Input: part model. Units: mm. Frame: model coordinates. Face numbers are marked on the shaded views. A direction names the side the tool comes from. Coordinates: 2 decimals unless noted, no trailing zeros. Loops run counter-clockwise (first coordinate to the right, second up) from the corner with the lowest first, then second, coordinate; pieces in that order, holes last. Notation, with made-up numbers: M -12,49 L 22,49 A28 ccw 22,76 Z; hole C 72,7 d7. An arc over 180 degrees is marked long. Use a Markdown table: item, result. Add a question column.
1. Line query: L1, parallel to Y at x = 21, z = 0; L2, parallel to Y at x = -31, z = -14; L3, parallel to Y at x = -2.5, z = 23.5. Output: solid intervals per line, ascending. Write a range as [from, to].
2. Draft query along Y for the marked faces 1, 2, 3 and 4. Return one class per face: +Y half, -Y half, draft (parallel to the pull), parting line (faces both ways), or undercut.
3. Set-up query: the marked faces 5 and 6. Return all of +Z, -Z, +X, -X, +Y, -Y with unobstructed straight access to the full face (end or side cutting, diameter ignored); none if empty.
4. Pin query (flat end, axial travel): pin 1 (1.5 mm diameter, centred on y = -3.5, z = -18.5, fed in from +X); pin 2 (4 mm diameter, centred on y = -24, z = 32, fed in from -X); pin 3 (10 mm diameter, centred on x = 6.5, y = 18.5, fed in from -Z). Return the tip coordinate at first contact, or that it passes through.
5. Section A-A on y = -14.5. Output: boundary loops of the cut face in (x, z).
6. Section C-C on x = -25.5. State how many separate pieces and enclosed holes the cut face has, then the cut area to 3 significant figures.
7. Section D-D on y = 6. Output: boundary loops of the cut face in (x, z), then the cut area to 3 significant figures.
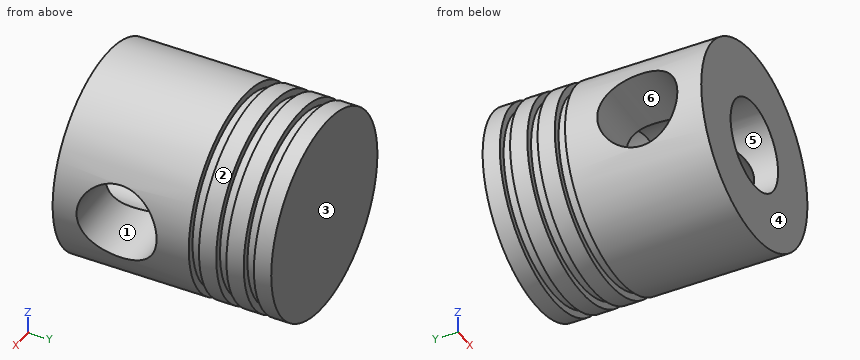
```python
from build123d import *

# Parameters (mm, degrees)
SKETCH4_R          = 16.9
CUT_EXTRUDE1_DEPTH = 42.5
SKETCH5_W          = 36
SKETCH5_H          = 40
SKETCH6_R          = 19
CUT_EXTRUDE2_DEPTH = 45


with BuildPart() as part:
    # Sketch2 → Revolve1 (revolve)
    with BuildSketch(Plane(origin=(0, 0, 0), x_dir=(0, 0, -1), z_dir=(1, 0, 0))):
        Polygon((39.5, 25.428946917), (39.5, 21.128946917), (42.5, 21.128946917), (42.5, 13.828946917), (39.5, 13.828946917), (39.5, 9.528946917), (42.5, 9.528946917), (42.5, -47.971053083), (0, -47.971053083), (0, 44.328946917), (42.5, 44.328946917), (42.5, 37.028946917), (39.5, 37.028946917), (39.5, 32.728946917), (42.5, 32.728946917), (42.5, 25.428946917), align=None)
    revolve(axis=Axis((0, -52.221053083, 0), (0, 1, 0)))

    # Sketch4 → Cut-Extrude1 (cut, symmetric)
    with BuildSketch(Plane(origin=(0, 0, 0), x_dir=(0, 0, -1), z_dir=(1, 0, 0))):
        with Locations((0, -20.971053083)):
            Circle(SKETCH4_R)
    extrude(amount=CUT_EXTRUDE1_DEPTH, both=True, mode=Mode.SUBTRACT)

    # Sketch5 → Cut-Revolve1 (revolve, cut)
    with BuildSketch(Plane(origin=(0, 0, 0), x_dir=(0, 0, -1), z_dir=(1, 0, 0))):
        with Locations((-18, 17.028946917)):
            Rectangle(SKETCH5_W, SKETCH5_H)
    revolve(axis=Axis((0, -52.221053083, 0), (0, 1, 0)), mode=Mode.SUBTRACT)

    # Sketch6 → Cut-Extrude2 (cut)
    with BuildSketch(Plane.XZ.offset(47.971053083)):
        Circle(SKETCH6_R)
    extrude(amount=-CUT_EXTRUDE2_DEPTH, mode=Mode.SUBTRACT)


solid = part.part
```
Answers below:
| question | item | result |
|---|---|---|
| 1 | L1 | y = [-47.97, -37.87], [-4.07, -2.97], [37.03, 44.33] |
| 1 | L2 | y = [-47.97, -30.44], [-11.5, -2.97], [37.03, 44.33] |
| 1 | L3 | y = [-47.97, -2.97], [37.03, 44.33] |
| 2 | face 1 | undercut |
| 2 | face 2 | draft |
| 2 | face 3 | +Y half |
| 2 | face 4 | -Y half |
| 3 | face 5 | -Y |
| 3 | face 6 | +X, -X |
| 4 | pin 1 | stops at x = 38.62 |
| 4 | pin 2 | stops at x = -30.1 |
| 4 | pin 3 | stops at z = -42.47 |
| 5 | outline | M -39.53,-15.61 A42.5 ccw 39.53,-15.61 L 10.83,-15.61 A19 cw -10.83,-15.61 Z; M -39.53,15.61 L -10.83,15.61 A19 cw 10.83,15.61 L 39.53,15.61 A42.5 ccw Z |
| 6 | separate pieces | 1 |
| 6 | enclosed holes | 2 |
| 6 | area | 3,250 mm² |
| 7 | outline | C 0,0 d85; hole C 0,0 d72 |
| 7 | area | 1,600 mm² |
